Check sheet for the modelled part. Datum: model origin and axes. Units: mm. Coordinates: 2 decimals unless noted, no trailing zeros. Write each loop counter-clockwise with the first axis right and the second up, starting at its lowest first coordinate (ties: lowest second). Pieces come first, ordered by that corner, then holes. Notation, with made-up numbers: (21.25, 10) -> (62.25, 10) arc R21 cw to (62.25, 33) -> close; hole circle Ø4 at (78.5, -28). An arc over 180 degrees is marked (long way). One line per item, written item: value. Start each with the question number.
1) Sectioned sample at B-B on y = 3.1. Give the number of separate pieces and of enclosed holes in the cut face, plus the area to 3 significant figures.
2) Draft check along Z on faces 1 (the cylindrical face through (58.62, 2.35, 0.68)), 2 (the flat face through (-1, 0, -1)), 3 (the cylindrical face through (-0.68, 2.35, 58.62)). Enter one of: +Z half, -Z half, draft (parallel to the pull), parting line (faces both ways), or undercut.
3) Sectioned sample at D-D on x = -18. Enter the section's corners in (y, z).
4) Sectioned sample at C-C on z = 33.02. Enter the section's corners in (x, y).
5) Scan lines: line 1 along Z through (x, y) = (50.8, 1.55); line 2 along Z through (x, y) = (-26.67, 2.65). Record each from-to range of solid material in increasing order. Write a range as [from, to].
6) Sectioned sample at A-A on x = 50.8. Enter the section's corners in (y, z), plus the area to 3 significant figures.
```python
from build123d import *

# Parameters (mm, degrees)
SKETCH1_R           = 4
SKETCH1_R_2         = 1.5875
BOSS_EXTRUDE1_DEPTH = 4.7625


with BuildPart() as part:
    # Sketch1 → Boss-Extrude1 (new body)
    with BuildSketch(Plane(origin=(0, 0, 0), x_dir=(1, 0, 0), z_dir=(0, 1, 0))):
        with BuildLine():
            ThreePointArc((-48.380952381, 63.267486058), (-59.780256121, 59.780256121), (-63.267486058, 48.380952381))
            ThreePointArc((-63.267486058, 48.380952381), (-58.617207227, 0), (-63.267486058, -48.380952381))
            ThreePointArc((-63.267486058, -48.380952381), (-59.780256121, -59.780256121), (-48.380952381, -63.267486058))
            ThreePointArc((-48.380952381, -63.267486058), (0, -58.617207227), (48.380952381, -63.267486058))
            ThreePointArc((48.380952381, -63.267486058), (59.780256121, -59.780256121), (63.267486058, -48.380952381))
            ThreePointArc((63.267486058, -48.380952381), (58.617207227, 0), (63.267486058, 48.380952381))
            ThreePointArc((63.267486058, 48.380952381), (59.780256121, 59.780256121), (48.380952381, 63.267486058))
            ThreePointArc((48.380952381, 63.267486058), (0, 58.617207227), (-48.380952381, 63.267486058))
        make_face()
        with Locations(Location((-50.8, 50.8, 0), (0, 0, 90))):
            Circle(SKETCH1_R, mode=Mode.SUBTRACT)
        with Locations(Location((50.8, 50.8, 0), (0, 0, 90))):
            Circle(SKETCH1_R, mode=Mode.SUBTRACT)
        with Locations(Location((50.8, -50.8, 0), (0, 0, 90))):
            Circle(SKETCH1_R, mode=Mode.SUBTRACT)
        with Locations(Location((-50.8, -50.8, 0), (0, 0, 90))):
            Circle(SKETCH1_R, mode=Mode.SUBTRACT)
        with Locations(Location((-26.67, 33.02, 0), (0, 0, 90))):
            Circle(SKETCH1_R_2, mode=Mode.SUBTRACT)
        with Locations(Location((26.67, 33.02, 0), (0, 0, 90))):
            Circle(SKETCH1_R_2, mode=Mode.SUBTRACT)
        with Locations(Location((-26.67, -33.02, 0), (0, 0, 90))):
            Circle(SKETCH1_R_2, mode=Mode.SUBTRACT)
        with Locations(Location((26.67, -33.02, 0), (0, 0, 90))):
            Circle(SKETCH1_R_2, mode=Mode.SUBTRACT)
    extrude(amount=BOSS_EXTRUDE1_DEPTH)


solid = part.part
```
Answers:
1. separate pieces: 1
1. enclosed holes: 8
1. area: 14,500 mm2
2. face 1: undercut
2. face 2: draft
2. face 3: +Z half
3. outline: (0, -59.26) -> (4.76, -59.26) -> (4.76, 59.26) -> (0, 59.26) -> close
4. outline: (-60.77, 0) -> (-28.26, 0) -> (-28.26, 4.76) -> (-60.77, 4.76) -> close; (-25.08, 0) -> (25.08, 0) -> (25.08, 4.76) -> (-25.08, 4.76) -> close; (28.26, 0) -> (60.77, 0) -> (60.77, 4.76) -> (28.26, 4.76) -> close
5. line 1: z = [-63.5, -54.8], [-46.8, 46.8], [54.8, 63.5]
5. line 2: z = [-60.02, -34.61], [-31.43, 31.43], [34.61, 60.02]
6. outline: (0, -63.5) -> (4.76, -63.5) -> (4.76, -54.8) -> (0, -54.8) -> close; (0, -46.8) -> (4.76, -46.8) -> (4.76, 46.8) -> (0, 46.8) -> close; (0, 54.8) -> (4.76, 54.8) -> (4.76, 63.5) -> (0, 63.5) -> close
6. area: 529 mm2
